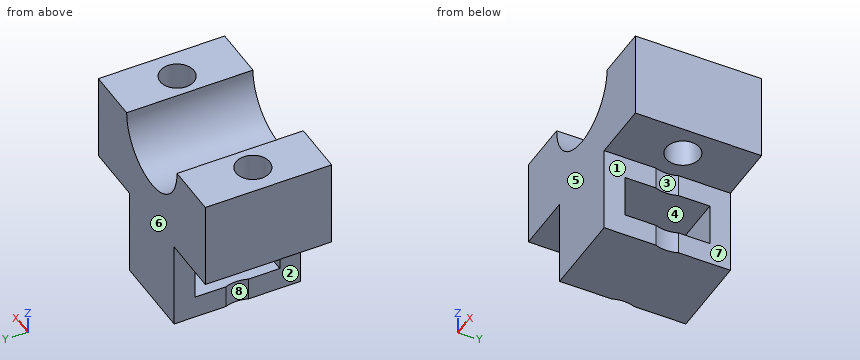
```python
from build123d import *

# Parameters (mm, degrees)
SKETCH_1_W          = 48
SKETCH_1_H          = 20
EXTRUDE_1_DEPTH     = 30
SKETCH_2_W          = 14
SKETCH_2_H          = 30
CUT_EXTRUDE_1_DEPTH = 7
SKETCH_7_W          = 22
SKETCH_7_H          = 30
EXTRUDE_2_DEPTH     = 48
SKETCH_8_W          = 21
SKETCH_8_H          = 30
CUT_EXTRUDE_2_DEPTH = 14
SKETCH_9_W          = 21
SKETCH_9_H          = 30
CUT_EXTRUDE_3_DEPTH = 14
SKETCH_11_W         = 10.2
SKETCH_11_H         = 20.2
CUT_EXTRUDE_4_DEPTH = 56.497747702
SKETCH_13_R         = 4
CUT_EXTRUDE_5_DEPTH = 44.783558558
SKETCH_14_R         = 4
CUT_EXTRUDE_6_DEPTH = 44.783558558
FILLET_1_R          = 7
SKETCH_20_R         = 7.5
CUT_EXTRUDE_8_DEPTH = 44.783558558
SKETCH2_R           = 11.3
CUT_EXTRUDE1_DEPTH  = 51


with BuildPart() as part:
    # Эскиз1 → Бобышка-Вытянуть1 (new body)
    with BuildSketch(Plane(origin=(0, 0, 0), x_dir=(1, 0, 0), z_dir=(0, 1, 0))):
        Rectangle(SKETCH_1_W, SKETCH_1_H)
    extrude(amount=EXTRUDE_1_DEPTH)

    # Эскиз2 → Вырез-Вытянуть1 (cut)
    with BuildSketch(Plane.XY.offset(10)):
        with Locations((0, 15)):
            Rectangle(SKETCH_2_W, SKETCH_2_H)
    extrude(amount=-CUT_EXTRUDE_1_DEPTH, mode=Mode.SUBTRACT)

    # Эскиз7 → Бобышка-Вытянуть2 (add)
    with BuildSketch(Plane(origin=(24, 0, 0), x_dir=(0, 0, -1), z_dir=(1, 0, 0))):
        with Locations((21, 15)):
            Rectangle(SKETCH_7_W, SKETCH_7_H)
    extrude(amount=-EXTRUDE_2_DEPTH)

    # Эскиз8 → Вырез-Вытянуть2 (cut)
    with BuildSketch(Plane(origin=(24, 0, 0), x_dir=(0, 0, -1), z_dir=(1, 0, 0))):
        with Locations((21.5, 15)):
            Rectangle(SKETCH_8_W, SKETCH_8_H)
    extrude(amount=-CUT_EXTRUDE_2_DEPTH, mode=Mode.SUBTRACT)

    # Эскиз9 → Вырез-Вытянуть3 (cut)
    with BuildSketch(Plane.ZY.offset(24)):
        with Locations((-21.5, 15)):
            Rectangle(SKETCH_9_W, SKETCH_9_H)
    extrude(amount=-CUT_EXTRUDE_3_DEPTH, mode=Mode.SUBTRACT)

    # Эскиз11 → Вырез-Вытянуть4 (cut, through all)
    with BuildSketch(Plane.ZY.offset(10)):
        with Locations((-21.5, 15)):
            Rectangle(SKETCH_11_W, SKETCH_11_H)
    extrude(amount=-CUT_EXTRUDE_4_DEPTH, mode=Mode.SUBTRACT)

    # Эскиз13 → Вырез-Вытянуть5 (cut, through all)
    with BuildSketch(Plane(origin=(0, 0, -11), x_dir=(-1, 0, 0), z_dir=(0, 0, -1))):
        with Locations((17, 15)):
            Circle(SKETCH_13_R)
    extrude(amount=-CUT_EXTRUDE_5_DEPTH, mode=Mode.SUBTRACT)

    # Эскиз14 → Вырез-Вытянуть6 (cut, through all)
    with BuildSketch(Plane(origin=(0, 0, -11), x_dir=(-1, 0, 0), z_dir=(0, 0, -1))):
        with Locations((-17, 15)):
            Circle(SKETCH_14_R)
    extrude(amount=-CUT_EXTRUDE_6_DEPTH, mode=Mode.SUBTRACT)

    # Скругление1
    fillet_1_edges = [part.edges().sort_by_distance(p)[0] for p in [
        (-7, 15, 3),
        (7, 15, 3),
    ]]
    fillet(fillet_1_edges, radius=FILLET_1_R - 0.0001)  # a hair under: the kernel refuses the full size

    # Эскиз20 → Вырез-Вытянуть8 (cut, through all)
    with BuildSketch(Plane(origin=(0, 0, -11), x_dir=(-1, 0, 0), z_dir=(0, 0, -1))):
        with Locations((-17, 15)):
            Circle(SKETCH_20_R)
        with Locations((17, 15)):
            Circle(SKETCH_20_R)
    extrude(amount=CUT_EXTRUDE_8_DEPTH, mode=Mode.SUBTRACT)

    # Sketch2 → Cut-Extrude1 (cut, through all)
    with BuildSketch(Plane(origin=(0, 30, 0), x_dir=(1, 0, 0), z_dir=(0, 1, 0))):
        with Locations((0, -10)):
            Circle(SKETCH2_R)
    extrude(amount=-CUT_EXTRUDE1_DEPTH, mode=Mode.SUBTRACT)


solid = part.part
```
Can you work these out from the model? Positions are in its coordinate system, mm. Face numbers are marked on the shaded views. A direction names the side the tool comes from. Coordinates: 2 decimals unless noted, no trailing zeros. Order: outer loops, then holes, each group sorted by start corner. A loop starts at its lowest first (then second) coordinate and runs counter-clockwise, first axis right, second up.
1. If we section it at A-A (y = 24.25): Please give me the cut outline in (x, z).
2. I need wall thicknesses on line 1 (X direction, y = 12.5, z = -8); line 2 (Y direction, x = -17, z = -6.5); line 3 (Y direction, x = 4, z = -21.5). Which ranges of each line are inside material? Lowest first, please.
3. For the marked faces 1, 2, 3 and 4, which set-ups out of +Z, -Z, +X, -X, +Y, -Y let a thin tool reach every point of the face, with its end or its side?
4. If we section it at C-C (x = 0): Please give me the cut outline in (y, z).
5. Thinking about a two-plate mould opening in Y: for the marked faces 5, 6, 7 and 8, which applies, +Y half, -Y half, draft (parallel to the pull), parting line (faces both ways), or undercut?
6. If we section it at D-D (x = 17): Please give me the cut outline in (y, z), then the cut area to 3 significant figures.
7. If we section it at B-B (z = 1.5): Please give me the cut outline in (x, y), then the cut area to 3 significant figures.
8. I'm going to push flat-ended pins straight in: pin 1 (8 mm diameter, centred on x = 15, y = 21.5, fed in from -Z); pin 2 (13.5 mm diameter, centred on y = 21, z = -23, fed in from -X); pin 3 (16 mm diameter, centred on x = -13.5, y = 16.5, fed in from -Z); pin 4 (13.5 mm diameter, centred on y = 21.5, z = -22, fed in from +X). Where does each tip first touch, or does it pass through?
Entries:
1. outline: (-24, -11) - (-10, -11) - (-10, -16.4) - (10, -16.4) - (10, -11) - (24, -11) - (24, 10) - (11.3, 10) arc R11.3 cw to (-11.3, 10) - (-24, 10) - close; (-10, -32) - (10, -32) - (10, -26.6) - (-10, -26.6) - close
2. line 1: x = -24 to -20.12, -13.88 to 13.88, 20.12 to 24
2. line 2: y = 0 to 11, 19 to 30
2. line 3: y = 0 to 4.9, 25.1 to 30
3. face 1: -Z, +X, +Y, -Y
3. face 2: -Z, -X, +Y, -Y
3. face 3: -Z, +X
3. face 4: +X, -X
4. outline: (0, -32) - (30, -32) - (30, -1.3) - (0, -1.3) - close; hole (4.9, -26.6) - (25.1, -26.6) - (25.1, -16.4) - (4.9, -16.4) - close
5. face 5: -Y half
5. face 6: +Y half
5. face 7: draft
5. face 8: undercut
6. outline: (0, -11) - (11, -11) - (11, 10) - (0, 10) - close; (19, -11) - (30, -11) - (30, 10) - (19, 10) - close
6. area: 462 mm2
7. outline: (-24, 0) - (-7.45, 0) - (-7.45, 30) - (-24, 30) - close; (7.45, 0) - (24, 0) - (24, 30) - (7.45, 30) - close; hole circle Ø8 at (-17, 15); hole circle Ø8 at (17, 15)
7. area: 893 mm2
8. pin 1: stops at z = -11
8. pin 2: stops at x = -10
8. pin 3: stops at z = -32
8. pin 4: stops at x = 10
